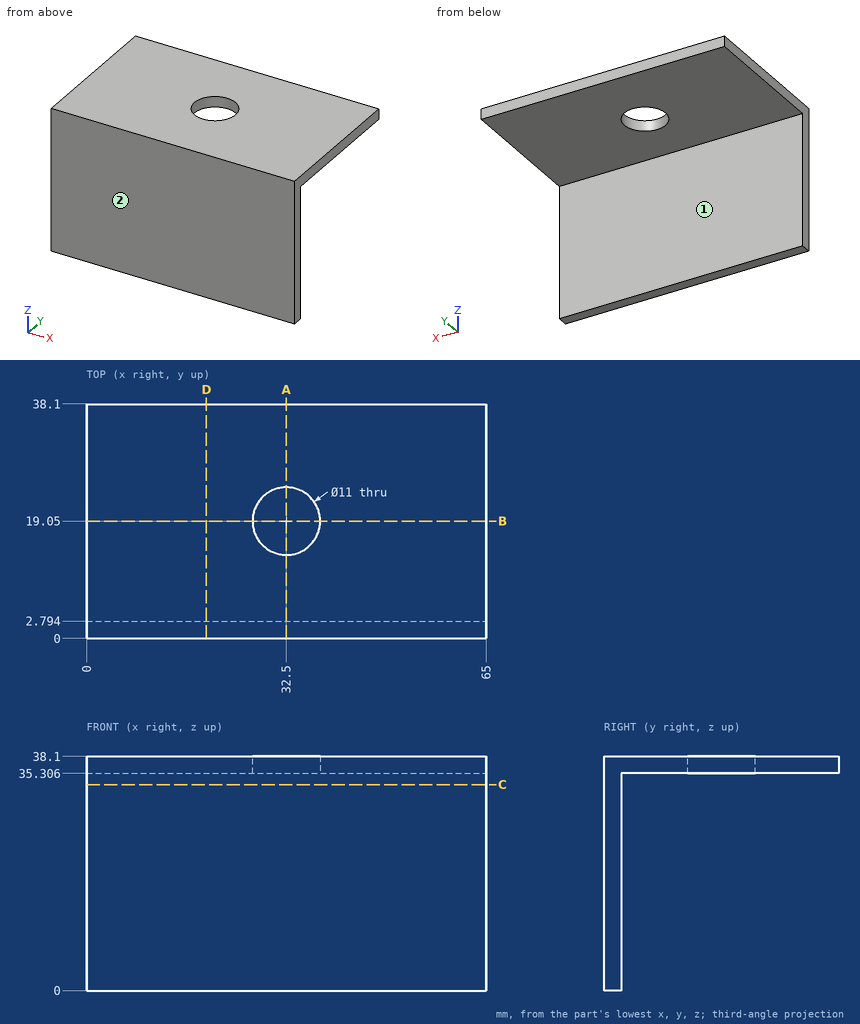
Verification items for this drawing (mm, ordinates from the low corner). A direction names the side the tool comes from. Round coordinates to 2 decimals unless told otherwise and drop trailing zeros. Loops run counter-clockwise (first coordinate to the right, second up) from the corner with the lowest first, then second, coordinate; pieces in that order, holes last. Notation, with made-up numbers: (2.25, 61) - (24.25, 61) arc R32 cw to (24.25, 95) - close; hole circle Ø7 at (-25.75, -30). An arc over 180 degrees is marked (long way). Answer as CSV lines item,"result". Start each with the question number.
Item 1: Section check C-C (z = 33.5). Record the boundary of the cut face in (x, y), and give its area (3 significant figures).
Item 2: Section check B-B (y = 19.05). Record the boundary of the cut face in (x, z).
Item 3: Section check D-D (x = 19.5). Record the boundary of the cut face in (y, z).
Item 4: Set-up check for the marked faces 1 and 2: record each of +Z, -Z, +X, -X, +Y, -Y from which the full face is reachable in a straight line by a thin tool's end or side.
Item 5: Section check A-A (x = 32.5). Record the boundary of the cut face in (y, z), and give its area (3 significant figures).
Item 6: Depth check by flat-ended pin: P1, Ø17.5, axis at x = 36, z = 18, coming from the +Y side; P2, Ø12, axis at x = 53, y = 29.5, coming from the -Z side; P3, Ø2, axis at x = 15, z = 4, coming from the -Y side. Enter the tip coordinate at first touch or a pass-through.
Item 7: Scan lines: line 1 (Y direction, x = 32.5, z = 36.65); line 2 (Y direction, x = 25, z = 32); line 3 (Z direction, x = 54, y = 32). Record each from-to range of solid material in increasing order. Write a range as [from, to].
Report:
1,outline,"(0, 0) - (65, 0) - (65, 2.79) - (0, 2.79) - close"
1,area,"182 mm2"
2,outline,"(0, 35.31) - (27, 35.31) - (27, 38.1) - (0, 38.1) - close; (38, 35.31) - (65, 35.31) - (65, 38.1) - (38, 38.1) - close"
3,outline,"(0, 0) - (2.79, 0) - (2.79, 35.31) - (38.1, 35.31) - (38.1, 38.1) - (0, 38.1) - close"
4,face 1,"-Z, +X, -X, +Y"
4,face 2,"+Z, -Z, +X, -X, -Y"
5,outline,"(0, 0) - (2.79, 0) - (2.79, 35.31) - (13.55, 35.31) - (13.55, 38.1) - (0, 38.1) - close; (24.55, 35.31) - (38.1, 35.31) - (38.1, 38.1) - (24.55, 38.1) - close"
5,area,"174 mm2"
6,P1,"stops at y = 2.79"
6,P2,"stops at z = 35.31"
6,P3,"stops at y = 0"
7,line 1,"y = [0, 13.55], [24.55, 38.1]"
7,line 2,"y = [0, 2.79]"
7,line 3,"z = [35.31, 38.1]"
